Input: part model. Units: mm. Frame: model coordinates. A direction names the side the tool comes from. Round coordinates to 2 decimals unless told otherwise and drop trailing zeros. Order: outer loops, then holes, each group sorted by start corner. A loop starts at its lowest first (then second) coordinate and runs counter-clockwise, first axis right, second up. Notation, with made-up numbers: (-18.5, 1) -> (33.5, 1) arc R30 cw to (33.5, 32) -> close; hole circle Ø7 at (-10, 73.25). An arc over 180 degrees is marked (long way). Use a Markdown table: item, result.
from build123d import *

# Parameters (mm, degrees)
SZKIC2_R                                = 6.5
DODANIE_WYCI_GNI_CIE1_DEPTH             = 219
DODANIE_WYCI_GNI_CIE1_DIRECTION_2_REACH = 38.742
SZKIC3_R                                = 4
DODANIE_WYCI_GNI_CIE2_DEPTH             = 16


with BuildPart() as part:
    # Szkic1 → Obrót5 (revolve)
    with BuildSketch(Plane.XY):
        with BuildLine():
            Line((0, 15), (0, -15))
            ThreePointArc((0, -15), (-15, 0), (0, 15))
        make_face()
    revolve(axis=Axis((0, 15, 0), (0, -1, 0)))

    # Szkic2 → Dodanie-wyciągnięcie1 (add)
    with BuildSketch(Plane(origin=(0, 0, -15), x_dir=(-1, 0, 0), z_dir=(0, 0, -1))):
        Circle(SZKIC2_R)
    extrude(amount=DODANIE_WYCI_GNI_CIE1_DEPTH)

    # Szkic2 → Dodanie-wyciągnięcie1 direction 2 (add, up to next)
    with BuildSketch(Plane(origin=(0, 0, -15), x_dir=(-1, 0, 0), z_dir=(0, 0, -1)), mode=Mode.PRIVATE) as dodanie_wyci_gni_cie1_direction_2_sk1:
        Circle(SZKIC2_R)
    dodanie_wyci_gni_cie1_direction_2_tool1 = extrude(dodanie_wyci_gni_cie1_direction_2_sk1.sketch, amount=-DODANIE_WYCI_GNI_CIE1_DIRECTION_2_REACH, mode=Mode.PRIVATE) - part.part
    add(dodanie_wyci_gni_cie1_direction_2_tool1.solids().sort_by_distance((0, 0, -15))[0])

    # Szkic3 → Dodanie-wyciągnięcie2 (add)
    with BuildSketch(Plane(origin=(0, 0, -234), x_dir=(-1, 0, 0), z_dir=(0, 0, -1))):
        Circle(SZKIC3_R)
    extrude(amount=DODANIE_WYCI_GNI_CIE2_DEPTH)


solid = part.part
1) Pull-direction query (Y, two-part tool) for faces 1 (the cylindrical face through (0.867, -3.905, -241.888)), 2 (the flat face through (-3, 3, -234)); classes: +Y half, -Y half, draft (parallel to the pull), parting line (faces both ways), or undercut.
Results found:
| item | result |
|---|---|
| face 1 | parting line |
| face 2 | draft |
2) Pin query (flat end, axial travel): pin 1 Ø10 at (y, z) = (11, -201) entering from +X; pin 2 Ø2 at (y, z) = (6, -19) entering from -X; pin 3 Ø1 at (y, z) = (1.5, -57) entering from -X. Return the tip coordinate at first contact, or that it passes through.
Results found:
| item | result |
|---|---|
| pin 1 | stops at x = 2.5 |
| pin 2 | stops at x = -4.15 |
| pin 3 | stops at x = -6.42 |
3) Cut plane A-A on y = 0. Return loops of the section in (x, z).
Results found:
| item | result |
|---|---|
| outline | (-6.5, -234) -> (-4, -234) -> (-4, -250) -> (4, -250) -> (4, -234) -> (6.5, -234) -> (6.5, -13.52) arc R15 ccw (long way) to (-6.5, -13.52) -> close |
4) Line query: L1, parallel to Y at x = -0.5, z = -39; L2, parallel to X at y = 9, z = -1.5; L3, parallel to Z at x = 12.25, y = -1.75. Output: solid intervals per line, ascending. Write a range as [from, to].
Results found:
| item | result |
|---|---|
| L1 | y = [-6.48, 6.48] |
| L2 | x = [-11.91, 11.91] |
| L3 | z = [-8.48, 8.48] |
5) Cut plane C-C on z = -82.5. Return loops of the section in (x, y), and give its area (3 significant figures).
Results found:
| item | result |
|---|---|
| outline | circle Ø13 at (0, 0) |
| area | 133 mm² |
6) Cut plane D-D on z = -4. Return loops of the section in (x, y), and give its area (3 significant figures).
Results found:
| item | result |
|---|---|
| outline | circle Ø28.91 at (0, 0) |
| area | 657 mm² |
7) Set-up query: faces 3 (the cylindrical face through (5.158, -3.955, -125.303)), 4 (the flat face through (0, 0, -250)). Return all of +Z, -Z, +X, -X, +Y, -Y with unobstructed straight access to the full face (end or side cutting, diameter ignored); none if empty.
Results found:
| item | result |
|---|---|
| face 3 | -Z |
| face 4 | -Z, +X, -X, +Y, -Y |
